```python
from build123d import *

# Parameters (mm, degrees)
SKETCH_1_R          = 11
EXTRUDE_1_DEPTH     = 2
SKETCH_2_R          = 5
EXTRUDE_2_DEPTH     = 10
SKETCH_3_R          = 1.5
CUT_EXTRUDE_1_DEPTH = 10
SKETCH_5_R          = 2
CUT_EXTRUDE_2_DEPTH = 20.646882704


with BuildPart() as part:
    # 草图1 → 凸台-拉伸1 (new body)
    with BuildSketch(Plane(origin=(0, 0, 0), x_dir=(0, 0, -1), z_dir=(0, 1, 0))):
        with Locations(Location((0, 0, 0), (0, 0, 180))):
            Circle(SKETCH_1_R)
    extrude(amount=EXTRUDE_1_DEPTH)

    # 草图2 → 凸台-拉伸2 (add)
    with BuildSketch(Plane(origin=(0, 2, 0), x_dir=(0, 0, -1), z_dir=(0, 1, 0))):
        with Locations(Location((0, 0, 0), (0, 0, 90))):
            Circle(SKETCH_2_R)
    extrude(amount=EXTRUDE_2_DEPTH)

    # 草图3 → 切除-拉伸1 (cut)
    with BuildSketch(Plane(origin=(0, 2, 0), x_dir=(0, 0, -1), z_dir=(0, 1, 0))):
        with Locations(Location((0, 8, 0), (0, 0, 90))):
            Circle(SKETCH_3_R)
        with Locations(Location((8.001, 0.001, 0), (0, 0, 90))):
            Circle(SKETCH_3_R)
        with Locations(Location((0.002, -8, 0), (0, 0, 90))):
            Circle(SKETCH_3_R)
        with Locations(Location((-7.999, -0.001, 0), (0, 0, 90))):
            Circle(SKETCH_3_R)
    extrude(amount=-CUT_EXTRUDE_1_DEPTH, mode=Mode.SUBTRACT)

    # 草图5 → 切除-拉伸2 (cut, through all)
    with BuildSketch(Plane(origin=(0, 12, 0), x_dir=(1, 0, 0), z_dir=(0, 1, 0))):
        with Locations(Location((0, 0, 0), (0, 0, 180))):
            Circle(SKETCH_5_R)
    extrude(amount=-CUT_EXTRUDE_2_DEPTH, mode=Mode.SUBTRACT)


solid = part.part
```
Input: part model. Units: mm. Frame: model coordinates. A direction names the side the tool comes from. Coordinates: 2 decimals unless noted, no trailing zeros. Loops run counter-clockwise (first coordinate to the right, second up) from the corner with the lowest first, then second, coordinate; pieces in that order, holes last. Notation, with made-up numbers: (-13, -37) - (5, -37) arc R30 cw to (5, -6) - close; hole circle Ø1 at (35.25, 63). An arc over 180 degrees is marked (long way). Answer in a Markdown table with one row per item.
(1) Cut plane D-D on x = 3.5. Output: boundary loops of the cut face in (y, z), plus the area to 3 significant figures.
Model answer:
| item | result |
|---|---|
| outline | (0, -10.43) - (2, -10.43) - (2, -3.57) - (12, -3.57) - (12, 3.57) - (2, 3.57) - (2, 10.43) - (0, 10.43) - close |
| area | 113 mm² |
(2) Cut plane A-A on z = 8.5. Output: boundary loops of the cut face in (x, y), plus the area to 3 significant figures.
Model answer:
| item | result |
|---|---|
| outline | (-6.98, 0) - (-1.41, 0) - (-1.41, 2) - (-6.98, 2) - close; (1.41, 0) - (6.98, 0) - (6.98, 2) - (1.41, 2) - close |
| area | 22.3 mm² |
(3) Cut plane B-B on x = -8. Output: boundary loops of the cut face in (y, z), plus the area to 3 significant figures.
Model answer:
| item | result |
|---|---|
| outline | (0, -7.55) - (2, -7.55) - (2, -1.5) - (0, -1.5) - close; (0, 1.5) - (2, 1.5) - (2, 7.55) - (0, 7.55) - close |
| area | 24.2 mm² |
(4) Material intervals for L1, parallel to X at y = 7, z = -1.25; L2, parallel to X at y = 7.75, z = -0.25; L3, parallel to Y at x = 6, z = -7.5, sorted ascending. Write a range as from..to.
Model answer:
| item | result |
|---|---|
| L1 | x = -4.84..-1.56, 1.56..4.84 |
| L2 | x = -4.99..-1.98, 1.98..4.99 |
| L3 | y = 0..2 |
(5) Pin query (flat end, axial travel): P1, Ø4, axis at x = -6.5, y = 8, coming from the +Z side; P2, Ø6, axis at x = -5, y = 6.5, coming from the -Z side; P3, Ø1.8, axis at x = -8, z = 0, coming from the +Y side; P4, Ø3, axis at x = -0.5, y = 4, coming from the +Z side. Return the tip coordinate at first contact, or that it passes through.
Model answer:
| item | result |
|---|---|
| P1 | stops at z = 2.18 |
| P2 | stops at z = -4.58 |
| P3 | passes through |
| P4 | stops at z = 5 |
(6) Mould query, pull axis X, two halves, no side actions, for faces 1 (the face through (-5, 2, 2)), 2 (the face through (-10.74, 0.99, -2.38)), 3 (the face through (9.5, 1.01, 0.06)). Classes: pulls with the +X half, pulls with the -X half, needs draft (parallel to the pull), parting line crosses it, or undercut.
Model answer:
| item | result |
|---|---|
| face 1 | needs draft |
| face 2 | parting line crosses it |
| face 3 | undercut |
(7) Set-up query: faces 4 (the face through (-2.2, 12, 0.1)), 5 (the face through (1.08, 6.93, -4.88)). Return all of +Z, -Z, +X, -X, +Y, -Y with unobstructed straight access to the full face (end or side cutting, diameter ignored); none if empty.
Model answer:
| item | result |
|---|---|
| face 4 | +Z, -Z, +X, -X, +Y |
| face 5 | +Y |
(8) Cut plane C-C on y = 3.5. Output: boundary loops of the cut face in (x, z).
Model answer:
| item | result |
|---|---|
| outline | circle Ø10 at (0, 0); hole circle Ø4 at (0, 0) |
